The listing builds one solid part. Answer for the finished solid, in the listing's coordinates (mm). Give positions to 0.01 mm unless a question says otherwise; leave off trailing zeros. Loops run counter-clockwise (first coordinate to the right, second up) from the corner with the lowest first, then second, coordinate; pieces in that order, holes last. Notation, with made-up numbers: (61.5, 35) - (112.5, 35) arc R26 ccw to (112.5, 55) - close; hole circle Ø4 at (-6, 3). An arc over 180 degrees is marked (long way). Answer as CSV lines item,"result". Start each with the question number.
1) A cutting plane is placed at D-D (z = 16). Determine the outline of the cut face in (x, y) (3 decimals).
2) A cutting plane is placed at B-B (x = -3.75). Determine the outline of the cut face in (y, z).
3) Flat-ended cylindrical pins translate along their axes: pin 1 (8 mm diameter, centred on x = -1.5, y = -12, fed in from +Z); pin 2 (3 mm diameter, centred on x = 4.5, y = -0.5, fed in from +Z); pin 3 (4 mm diameter, centred on x = -6.5, y = -13.5, fed in from +Z); pin 4 (1.5 mm diameter, centred on x = 3.5, z = 9.5, fed in from -Y). Find the tip coordinate at first contact, or state that the pin passes through.
4) A cutting plane is placed at C-C (y = -7.5). Determine the outline of the cut face in (x, z) (3 decimals).
5) Find the intervals of material crossed by line 1 along Z through (x, y) = (4, 0); line 2 along Y through (x, z) = (3, -11); line 3 along Z through (x, y) = (5.5, 2), in increasing order.
6) A cutting plane is placed at A-A (z = 0). Determine the outline of the cut face in (x, y) (3 decimals), and give its area (3 significant figures).
7) For a pull along Z with two mould halves and no side action, classify faces 1 (the face through (0, 16, 25.4)), 2 (the face through (-0.13, -2.75, -12.4)), 3 (the face through (0, 31.75, 0)) as pulls with the +Z half, pulls with the -Z half, needs draft (parallel to the pull), parting line crosses it, or undercut.
```python
from build123d import *

# Parameters (mm, degrees)
F0_R     = 12.7
F1_DEPTH = 9.525


with BuildPart() as f1:
    # F0 (on Right) → F1 (new body, symmetric)
    with BuildSketch(Plane.YZ):
        with BuildLine():
            Line((31.75, 25.4), (0, 25.4))
            ThreePointArc((0, 25.4), (-25.4, 0), (0, -25.4))
            Line((0, -25.4), (31.75, -25.4))
            Line((31.75, -25.4), (31.75, 25.4))
        make_face()
        Circle(F0_R, mode=Mode.SUBTRACT)
    extrude(amount=F1_DEPTH, both=True)


solid = f1.part
```
Ans:
1,outline,"(-9.525, -19.727) - (9.525, -19.727) - (9.525, 31.75) - (-9.525, 31.75) - close"
2,outline,"(0, -25.4) - (31.75, -25.4) - (31.75, 25.4) - (0, 25.4) arc R25.4 ccw to start; hole circle Ø25.4 at (0, 0)"
3,pin 1,"z = 24.11"
3,pin 2,"z = 25.4"
3,pin 3,"z = 22.65"
3,pin 4,"y = -23.85"
4,outline,"(-9.525, -24.267) - (9.525, -24.267) - (9.525, -10.249) - (-9.525, -10.249) - close; (-9.525, 10.249) - (9.525, 10.249) - (9.525, 24.267) - (-9.525, 24.267) - close"
5,line 1,"-25.4 to -12.7, 12.7 to 25.4"
5,line 2,"-22.89 to -6.35, 6.35 to 31.75"
5,line 3,"-25.4 to -12.54, 12.54 to 25.4"
6,outline,"(-9.525, -25.4) - (9.525, -25.4) - (9.525, -12.7) - (-9.525, -12.7) - close; (-9.525, 12.7) - (9.525, 12.7) - (9.525, 31.75) - (-9.525, 31.75) - close"
6,area,"605 mm2"
7,face 1,"pulls with the +Z half"
7,face 2,"undercut"
7,face 3,"needs draft"
